```python
from build123d import *

# Parameters (mm, degrees)
F0_W     = 2.9037779868
F0_H     = 66.5
F1_DEPTH = 2.5
F2_DEPTH = 9.33
F3_R     = 1.1
F4_DEPTH = 3.25


# Not quite as in the source:
# - a feature names something its author has since deleted; it is built from what else it names


with BuildPart() as f1:
    # F0 (on Front) → F1 (new body)
    with BuildSketch(Plane.XZ):
        with Locations((-24.4931335896, -18.415993683)):
            Rectangle(F0_W, F0_H)
        Polygon((-20.845022583, 14.834006317), (-23.0412445962, 14.834006317), (-23.0412445962, -51.665993683), (-17.345022583, -51.665993683), (-17.345022583, 14.834006317), align=None)
    extrude(amount=F1_DEPTH)

    # F0 (on Front) → F2, piece 2 (join)
    with BuildSketch(Plane.XZ):
        Polygon((-20.845022583, 14.834006317), (-23.0412445962, 14.834006317), (-23.0412445962, -51.665993683), (-17.345022583, -51.665993683), (-17.345022583, 14.834006317), align=None)
    extrude(amount=-F2_DEPTH)



with BuildPart() as f1b:
    # F0 (on Front) → F1, piece 2 (new body)
    with BuildSketch(Plane.XZ):
        with Locations((76.6030884236, -18.415993683)):
            Rectangle(F0_W, F0_H)
        Polygon((72.954977417, 14.834006317), (69.454977417, 14.834006317), (69.454977417, -51.665993683), (75.1511994302, -51.665993683), (75.1511994302, 14.834006317), align=None)
    extrude(amount=F1_DEPTH)

    # F0 (on Front) → F2 (join)
    with BuildSketch(Plane.XZ):
        Polygon((72.954977417, 14.834006317), (69.454977417, 14.834006317), (69.454977417, -51.665993683), (75.1511994302, -51.665993683), (75.1511994302, 14.834006317), align=None)
    extrude(amount=-F2_DEPTH)


with BuildPart() as f1_1:
    add(f1.part)

    add(f1b.part)  # F4 merges F1b
    # F3 (on face) → F4 (join)
    with BuildSketch(Plane(origin=(0, 9.33, 0), x_dir=(-1, 0, 0), z_dir=(0, 1, 0))):
        Polygon((17.345022583, -51.665993683), (17.345022583, 14.834006317), (7.945022583, 14.834006317), (-26.054977417, 14.834006317), (-60.054977417, 14.834006317), (-75.1511994302, 14.834006317), (-75.1511994302, -51.665993683), align=None)
        with Locations((-64.854977417, -42.165993683)):
            Circle(F3_R, mode=Mode.SUBTRACT)
        with Locations((12.745022583, -42.165993683)):
            Circle(F3_R, mode=Mode.SUBTRACT)
        Polygon((-26.054977417, 14.834006317), (7.945022583, 14.834006317), (-9.554977417, 73.334006317), (-26.054977417, 73.334006317), (-42.554977417, 73.334006317), (-60.054977417, 14.834006317), align=None)
        with Locations((-26.054977417, 63.584006317)):
            Circle(F3_R, mode=Mode.SUBTRACT)
    extrude(amount=-F4_DEPTH)


solid = f1_1.part
```
Design review of the part built by this model. Coordinates are the model's own, in mm. A direction names the side the tool comes from. Give positions to 0.01 mm unless a question says otherwise; leave off trailing zeros. Write each loop counter-clockwise with the first axis right and the second up, starting at its lowest first coordinate (ties: lowest second). Pieces come first, ordered by that corner, then holes. Notation, with made-up numbers: (79, 40.25) -> (90, 40.25) arc R24 cw to (90, 60.25) -> close; hole circle Ø9 at (38.5, -21). An arc over 180 degrees is marked (long way). Answer in a Markdown table with one row per item.
(1) Clearance check with flat-ended pins moving along their axes: pin 1 (1.8 mm diameter, centred on x = 26.05, z = 63.58, fed in from -Y); pin 2 (3 mm diameter, centred on x = 13.5, z = -14, fed in from -Y); pin 3 (2.5 mm diameter, centred on x = 76.5, z = -19.5, fed in from +Y); pin 4 (5 mm diameter, centred on y = 4.5, z = -15, fed in from -X). State where each tip first meets the part, or that it passes through.
Results:
| item | result |
|---|---|
| pin 1 | through |
| pin 2 | y = 6.08 |
| pin 3 | y = 0 |
| pin 4 | x = -23.04 |
(2) Consider section D-D (z = 36). State the section outline as (x, y) points, then the cut area to 3 significant figures.
Results:
| item | result |
|---|---|
| outline | (-1.61, 6.08) -> (53.72, 6.08) -> (53.72, 9.33) -> (-1.61, 9.33) -> close |
| area | 180 mm2 |
(3) Consider section C-C (x = 13.5). State the section outline as (y, z) points, then the cut area to 3 significant figures.
Results:
| item | result |
|---|---|
| outline | (6.08, -51.67) -> (9.33, -51.67) -> (9.33, 73.33) -> (6.08, 73.33) -> close |
| area | 406 mm2 |
(4) For faces 1 (the flat face through (71, 5, 14.834)), 2 (the flat face through (-19, 5, 14.834)), 3 (the flat face through (-17.345, 2, -19)), list the 3-axis set-ups (+Z, -Z, +X, -X, +Y, -Y) from which the entire face can be reached by the end or side of a thin tool; tool diameter is ignored.
Results:
| item | result |
|---|---|
| face 1 | +Z, +X, +Y, -Y |
| face 2 | +Z, -X, +Y, -Y |
| face 3 | +Z, -Z, -Y |
(5) Consider section B-B (z = -38.5). State the section outline as (x, y) points.
Results:
| item | result |
|---|---|
| outline | (-25.95, -2.5) -> (-17.35, -2.5) -> (-17.35, 6.08) -> (69.45, 6.08) -> (69.45, -2.5) -> (78.05, -2.5) -> (78.05, 0) -> (75.15, 0) -> (75.15, 9.33) -> (-23.04, 9.33) -> (-23.04, 0) -> (-25.95, 0) -> close |
(6) To check wall thickness, follow probe 1 along X at (y, z) = (3, 7); probe 2 along Y at (x, z) = (49, 6.5); probe 3 along X at (y, z) = (8.75, -31). State the ranges of each line that lie inside material, in increasing order.
Results:
| item | result |
|---|---|
| probe 1 | -23.04 to -17.35, 69.45 to 75.15 |
| probe 2 | 6.08 to 9.33 |
| probe 3 | -23.04 to 75.15 |
(7) Consider section A-A (y = 3.5). State the section outline as (x, z) points.
Results:
| item | result |
|---|---|
| outline | (-23.04, -51.67) -> (-17.35, -51.67) -> (-17.35, 14.83) -> (-23.04, 14.83) -> close; (69.45, -51.67) -> (75.15, -51.67) -> (75.15, 14.83) -> (69.45, 14.83) -> close |
(8) Mouldability with a two-part tool opening along X and no side actions: class faces 4 (the flat face through (-25, 0, -18)), 5 (the flat face through (27, 6.08, -2)), 6 (the flat face through (69.455, 2, -18)), 7 (the flat face through (-23.041, 5, -18)) as +X half, -X half, draft (parallel to the pull), parting line (faces both ways), or undercut.
Results:
| item | result |
|---|---|
| face 4 | draft |
| face 5 | undercut |
| face 6 | undercut |
| face 7 | -X half |
